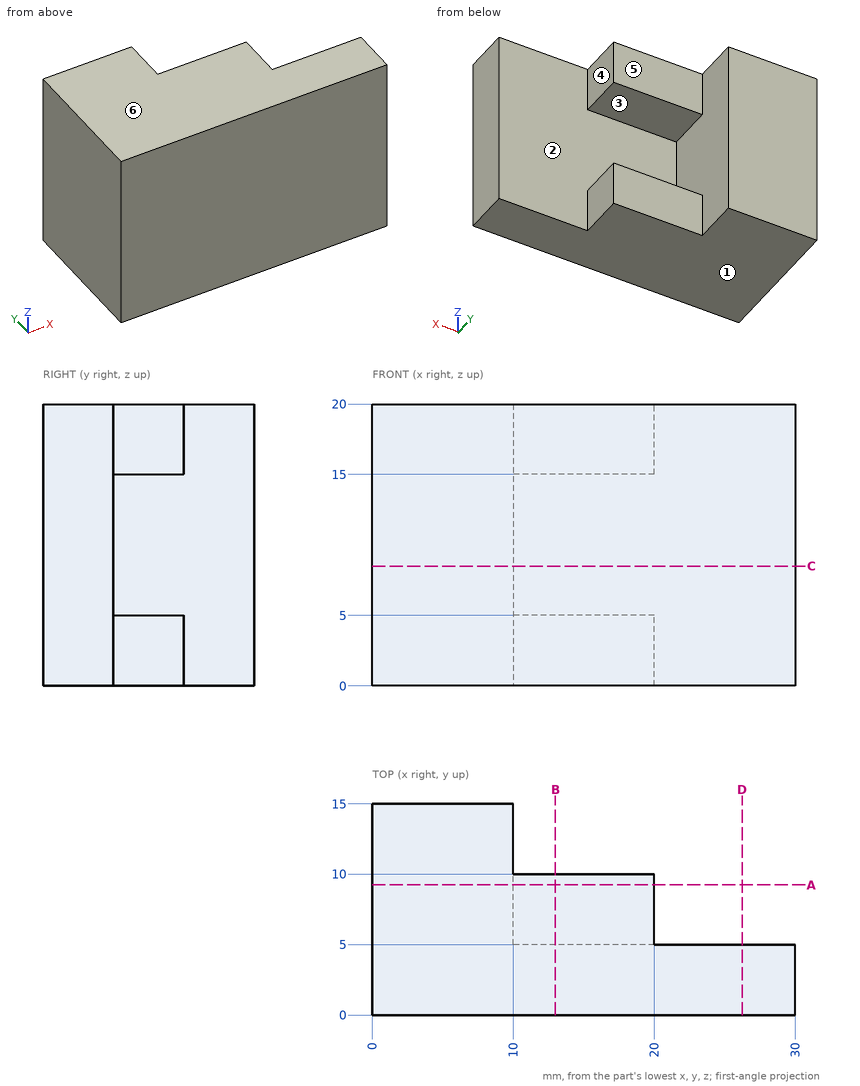
Answer from the drawing. Dimensions are ordinates in mm from the lowest x, y and z of the part. A direction names the side the tool comes from. Coordinates: 2 decimals unless noted, no trailing zeros. Order: outer loops, then holes, each group sorted by start corner. A loop starts at its lowest first (then second) coordinate and runs counter-clockwise, first axis right, second up. Notation, with made-up numbers: (-37, -21) -> (1, -21) arc R19 ccw to (1, 10) -> close; hole circle Ø5 at (19.25, -19). An arc over 180 degrees is marked (long way). Answer as a JSON object with one key per item and string values.
1) The mould has two halves that part along Z. Classify the marked faces 1, 2, 3 and 4: released by +Z, released by -Z, zero draft, split by the parting line, or undercut.
Model answer:
{"face 1": "released by -Z", "face 2": "undercut", "face 3": "undercut", "face 4": "zero draft"}
2) A cutting plane is placed at A-A, the plane y = 9.25. Determine the outline of the cut face in (x, z).
Model answer:
{"outline": "(0, 0) -> (20, 0) -> (20, 5) -> (10, 5) -> (10, 15) -> (20, 15) -> (20, 20) -> (0, 20) -> close"}
3) A cutting plane is placed at D-D, the plane x = 26.25. Determine the outline of the cut face in (y, z).
Model answer:
{"outline": "(0, 0) -> (5, 0) -> (5, 20) -> (0, 20) -> close"}
4) A cutting plane is placed at B-B, the plane x = 13. Determine the outline of the cut face in (y, z), plus the area to 3 significant figures.
Model answer:
{"outline": "(0, 0) -> (10, 0) -> (10, 5) -> (5, 5) -> (5, 15) -> (10, 15) -> (10, 20) -> (0, 20) -> close", "area": "150 mm²"}
5) A cutting plane is placed at C-C, the plane z = 8.5. Determine the outline of the cut face in (x, y), plus the area to 3 significant figures.
Model answer:
{"outline": "(0, 0) -> (30, 0) -> (30, 5) -> (10, 5) -> (10, 15) -> (0, 15) -> close", "area": "250 mm²"}
6) Each of these flat-tipped pins is pushed along its axis until it touches: pin 1 (1.5 mm diameter, centred on x = 13.5, z = 2.5, fed in from +Y); pin 2 (5 mm diameter, centred on y = 12, z = 2.5, fed in from -X); pin 3 (5.5 mm diameter, centred on y = 8, z = 18, fed in from +X); pin 4 (1 mm diameter, centred on x = 21, y = 8, fed in from -Z). Where does it stop, or does it pass through?
Model answer:
{"pin 1": "stops at y = 10", "pin 2": "stops at x = 0", "pin 3": "stops at x = 20", "pin 4": "passes through"}
7) A tool of negligible diameter and unlimited length cuts with its end or side. For the marked faces 5 and 6, from which of +Z, -Z, +X, -X, +Y, -Y can it reach the whole face along a straight path? Write none if from no direction.
Model answer:
{"face 5": "+Z, -Z, +X, +Y", "face 6": "+Z, +X, -X, +Y, -Y"}
8) Consider line 1 along Y through (x, z) = (24.75, 14.25); line 2 along Y through (x, z) = (14.25, 18.5). Determine where each line is inside the solid, lowest interval first. Write a range as from..to.
Model answer:
{"line 1": "y = 0..5", "line 2": "y = 0..10"}
